from build123d import *

# Parameters (mm, degrees)
SKETCH1_W                = 55
SKETCH1_H                = 80
BACKPANEL_DEPTH          = 3
SKETCH2_W                = 7.325
SKETCH2_H                = 4
MOTORMOUNT_DEPTH         = 34
SKETCH3_W                = 37
SKETCH3_H                = 80
SIDEPANEL2_DEPTH         = 3
SKETCH4_W                = 37
SKETCH4_H                = 80
SIDEPANEL1_DEPTH         = 3
MOTORSUPPORTANGLES_DEPTH = 34
MOTORHOLESSET1_REACH     = 92.957
SKETCH5_R                = 1.515
MOTORHOLESSET2_REACH     = 92.957
SKETCH5_3_R              = 1.515
SKETCH7_W                = 61
SKETCH7_H                = 37
BOTTOMPLATE_DEPTH        = 3
SKETCH8_W                = 61
SKETCH8_H                = 3
CUT_EXTRUDE1_DEPTH       = 37
SKETCH20_W               = 100.196149356
SKETCH20_H               = 67.738241818
SKETCH20_R               = 2
BOSS_EXTRUDE8_DEPTH      = 20
BOSS_EXTRUDE10_DEPTH     = 10
BOSS_EXTRUDE11_DEPTH     = 8
SKETCH24_R               = 1.505
CUT_EXTRUDE6_DEPTH       = 4
SKETCH25_W               = 7.25
SKETCH25_H               = 7.25
BOSS_EXTRUDE12_DEPTH     = 7.25
SKETCH26_R               = 1.515
CUT_EXTRUDE7_DEPTH       = 7.25
CUT_EXTRUDE8_REACH       = 113.941
SKETCH27_W               = 7.325
SKETCH27_H               = 4.500198619
FILLET3_R                = 4.5
SKETCH28_W               = 55
SKETCH28_H               = 16.687272165
CUT_EXTRUDE9_DEPTH       = 3
SKETCH30_W               = 100.196149356
SKETCH30_H               = 67.738241818
CUT_EXTRUDE10_DEPTH      = 10
CHAMFER1_SIZE            = 10
CHAMFER2_SIZE            = 10
CHAMFER3_SIZE            = 10
SKETCH31_R               = 3.5
CUT_EXTRUDE11_DEPTH      = 10
SKETCH32_W               = 49.142704434
SKETCH32_H               = 21.220713278
CUT_EXTRUDE12_DEPTH      = 10
SKETCH33_W               = 25.755482036
SKETCH33_H               = 3
CUT_EXTRUDE13_DEPTH      = 10


with BuildPart() as part:
    # Sketch1 → BackPanel (new body)
    with BuildSketch(Plane.XY):
        with Locations((27.5, 40)):
            Rectangle(SKETCH1_W, SKETCH1_H)
    extrude(amount=BACKPANEL_DEPTH)

    # Sketch2 → MotorMount (add)
    with BuildSketch(Plane.XY.offset(3)):
        with Locations((3.6625, 18.5)):
            Rectangle(SKETCH2_W, SKETCH2_H)
        with Locations((51.3375, 18.5)):
            Rectangle(SKETCH2_W, SKETCH2_H)
    extrude(amount=MOTORMOUNT_DEPTH)

    # Sketch3 → SidePanel2 (add)
    with BuildSketch(Plane.ZY):
        with Locations((18.5, 40)):
            Rectangle(SKETCH3_W, SKETCH3_H)
    extrude(amount=SIDEPANEL2_DEPTH)

    # Sketch4 → SidePanel1 (add)
    with BuildSketch(Plane(origin=(55, 0, 0), x_dir=(0, 0, -1), z_dir=(1, 0, 0))):
        with Locations((-18.5, 40)):
            Rectangle(SKETCH4_W, SKETCH4_H)
    extrude(amount=SIDEPANEL1_DEPTH)

    # Sketch6 → MotorSupportAngles (add)
    with BuildSketch(Plane.XY.offset(37)):
        Polygon((7.325, 16.5), (0, 3.812727835), (0, 16.5), align=None)
        Polygon((47.675, 16.5), (55, 16.5), (55, 3.812727835), align=None)
    extrude(amount=-MOTORSUPPORTANGLES_DEPTH)

    # MotorHolesSet1: up to this plane
    motorholesset1_end = Plane(origin=(7.325, 16.5, -11.65), z_dir=(0.866025403784438, -0.5000000000000012, 0))
    # Sketch5 → MotorHolesSet1 (cut, up to the surface)
    with BuildSketch(Plane(origin=(0, 20.5, 0), x_dir=(1, 0, 0), z_dir=(0, 1, 0)), mode=Mode.PRIVATE) as motorholesset1_sk1:
        with Locations(Location((3.2, -15.1, 0), (0, 0, 270))):
            Circle(SKETCH5_R)
    motorholesset1_tool1 = split(extrude(motorholesset1_sk1.sketch, amount=-MOTORHOLESSET1_REACH, mode=Mode.PRIVATE), bisect_by=motorholesset1_end, keep=Keep.BOTH, mode=Mode.PRIVATE)
    add(motorholesset1_tool1.solids().sort_by_distance((3.2, 20.5, 15.1))[0], mode=Mode.SUBTRACT)
    # Sketch5 → MotorHolesSet1 (cut, up to the surface)
    with BuildSketch(Plane(origin=(0, 20.5, 0), x_dir=(1, 0, 0), z_dir=(0, 1, 0)), mode=Mode.PRIVATE) as motorholesset1_sk2:
        with Locations(Location((3.2, -24.9, 0), (0, 0, 270))):
            Circle(SKETCH5_R)
    motorholesset1_tool2 = split(extrude(motorholesset1_sk2.sketch, amount=-MOTORHOLESSET1_REACH, mode=Mode.PRIVATE), bisect_by=motorholesset1_end, keep=Keep.BOTH, mode=Mode.PRIVATE)
    add(motorholesset1_tool2.solids().sort_by_distance((3.2, 20.5, 24.9))[0], mode=Mode.SUBTRACT)

    # MotorHolesSet2: up to this plane
    motorholesset2_end = Plane(origin=(55, 3.812727835, -11.65), z_dir=(-0.866025403784438, -0.5000000000000011, 0))
    # Sketch5<3> → MotorHolesSet2 (cut, up to the surface)
    with BuildSketch(Plane(origin=(0, 20.5, 0), x_dir=(1, 0, 0), z_dir=(0, 1, 0)), mode=Mode.PRIVATE) as motorholesset2_sk1:
        with Locations(Location((51.8, -15.1, 0), (0, 0, 270))):
            Circle(SKETCH5_3_R)
    motorholesset2_tool1 = split(extrude(motorholesset2_sk1.sketch, amount=-MOTORHOLESSET2_REACH, mode=Mode.PRIVATE), bisect_by=motorholesset2_end, keep=Keep.BOTH, mode=Mode.PRIVATE)
    add(motorholesset2_tool1.solids().sort_by_distance((51.8, 20.5, 15.1))[0], mode=Mode.SUBTRACT)
    # Sketch5<3> → MotorHolesSet2 (cut, up to the surface)
    with BuildSketch(Plane(origin=(0, 20.5, 0), x_dir=(1, 0, 0), z_dir=(0, 1, 0)), mode=Mode.PRIVATE) as motorholesset2_sk2:
        with Locations(Location((51.8, -24.9, 0), (0, 0, 270))):
            Circle(SKETCH5_3_R)
    motorholesset2_tool2 = split(extrude(motorholesset2_sk2.sketch, amount=-MOTORHOLESSET2_REACH, mode=Mode.PRIVATE), bisect_by=motorholesset2_end, keep=Keep.BOTH, mode=Mode.PRIVATE)
    add(motorholesset2_tool2.solids().sort_by_distance((51.8, 20.5, 24.9))[0], mode=Mode.SUBTRACT)

    # Sketch7 → BottomPlate (add)
    with BuildSketch(Plane.XZ):
        with Locations((27.5, 18.5)):
            Rectangle(SKETCH7_W, SKETCH7_H)
    extrude(amount=BOTTOMPLATE_DEPTH)

    # Sketch8 → Cut-Extrude1 (cut)
    with BuildSketch(Plane.XY.offset(37)):
        with Locations((27.5, -1.5)):
            Rectangle(SKETCH8_W, SKETCH8_H)
    extrude(amount=-CUT_EXTRUDE1_DEPTH, mode=Mode.SUBTRACT)



with BuildPart() as body_2:
    # Sketch20 → Boss-Extrude8 (new body)
    with BuildSketch(Plane(origin=(0, -30, 0), x_dir=(-1, 0, 0), z_dir=(0, -1, 0))):
        with Locations((-27.5, -20.61971831)):
            Rectangle(SKETCH20_W, SKETCH20_H)
        with Locations(Location((8, -44.61971831, 0), (0, 0, 90))):
            Circle(SKETCH20_R, mode=Mode.SUBTRACT)
        with Locations(Location((-63, -44.61971831, 0), (0, 0, 90))):
            Circle(SKETCH20_R, mode=Mode.SUBTRACT)
        with Locations(Location((-63, 3.38028169, 0), (0, 0, 90))):
            Circle(SKETCH20_R, mode=Mode.SUBTRACT)
        with Locations(Location((8, 3.38028169, 0), (0, 0, 90))):
            Circle(SKETCH20_R, mode=Mode.SUBTRACT)
    extrude(amount=-BOSS_EXTRUDE8_DEPTH)


with BuildPart() as part_1:
    add(part.part)

    add(body_2.part)  # Boss-Extrude10 merges body 2
    # Sketch21 → Boss-Extrude10 (add)
    with BuildSketch(Plane.XZ):
        Polygon((-3, 0), (58, 0), (58, 37), (55, 37), (55, 3), (0, 3), (0, 37), (-3, 37), align=None)
    extrude(amount=BOSS_EXTRUDE10_DEPTH)

    # Sketch22 → Boss-Extrude11 (add)
    with BuildSketch(Plane.XY.offset(3)):
        Polygon((0, 76.85), (7, 76.85), (7, 73.35), (0, 66.35), align=None)
        Polygon((55, 76.85), (55, 66.35), (48, 73.35), (48, 76.85), align=None)
    extrude(amount=BOSS_EXTRUDE11_DEPTH)

    # Sketch24 → Cut-Extrude6 (cut)
    with BuildSketch(Plane(origin=(0, 76.85, 0), x_dir=(1, 0, 0), z_dir=(0, 1, 0))):
        with Locations(Location((3.5, -7, 0), (0, 0, 180))):
            Circle(SKETCH24_R)
        with Locations(Location((51.5, -7, 0), (0, 0, 180))):
            Circle(SKETCH24_R)
    extrude(amount=-CUT_EXTRUDE6_DEPTH, mode=Mode.SUBTRACT)

    # Sketch25 → Boss-Extrude12 (add)
    with BuildSketch(Plane(origin=(0, -10, 0), x_dir=(1, 0, 0), z_dir=(0, 1, 0))):
        with Locations((3.625, -30.375)):
            Rectangle(SKETCH25_W, SKETCH25_H)
        with Locations((51.375, -30.375)):
            Rectangle(SKETCH25_W, SKETCH25_H)
    extrude(amount=BOSS_EXTRUDE12_DEPTH)

    # Sketch26 → Cut-Extrude7 (cut)
    with BuildSketch(Plane.XY.offset(34)):
        with Locations((3.625, -6.375)):
            Circle(SKETCH26_R)
        with Locations((51.375, -6.375)):
            Circle(SKETCH26_R)
    extrude(amount=-CUT_EXTRUDE7_DEPTH, mode=Mode.SUBTRACT)

    # Cut-Extrude8: up to this plane
    cut_extrude8_end = Plane(origin=(7.325, 16.5, -11.65), z_dir=(0.866025403784438, -0.5000000000000012, 0))
    # Sketch27 → Cut-Extrude8 (cut, up to the surface)
    with BuildSketch(Plane(origin=(0, 20.5, 0), x_dir=(1, 0, 0), z_dir=(0, 1, 0)), mode=Mode.PRIVATE) as cut_extrude8_sk1:
        with Locations((3.6625, -19.611135977)):
            Rectangle(SKETCH27_W, SKETCH27_H)
    cut_extrude8_tool1 = split(extrude(cut_extrude8_sk1.sketch, amount=-CUT_EXTRUDE8_REACH, mode=Mode.PRIVATE), bisect_by=cut_extrude8_end, keep=Keep.BOTH, mode=Mode.PRIVATE)
    add(cut_extrude8_tool1.solids().sort_by_distance((3.6625, 20.5, 19.611136))[0], mode=Mode.SUBTRACT)

    # Fillet3
    fillet3_edges = [part_1.edges().sort_by_distance(p)[0] for p in [
        (48, 75.1, 11),
    ]]
    fillet(fillet3_edges, radius=FILLET3_R)

    # Sketch28 → Cut-Extrude9 (cut)
    with BuildSketch(Plane.XY.offset(37)):
        with Locations((27.5, 12.156363918)):
            Rectangle(SKETCH28_W, SKETCH28_H)
    extrude(amount=-CUT_EXTRUDE9_DEPTH, mode=Mode.SUBTRACT)

    # Sketch30 → Cut-Extrude10 (cut)
    with BuildSketch(Plane.XZ.offset(30)):
        with Locations((27.5, 20.61971831)):
            Rectangle(SKETCH30_W, SKETCH30_H)
    extrude(amount=-CUT_EXTRUDE10_DEPTH, mode=Mode.SUBTRACT)

    # Chamfer1
    chamfer1_edges = [part_1.edges().sort_by_distance(p)[0] for p in [
        (-3, -10, 18.5),
    ]]
    chamfer(chamfer1_edges, length=CHAMFER1_SIZE)

    # Chamfer2
    chamfer2_edges = [part_1.edges().sort_by_distance(p)[0] for p in [
        (58, -10, 18.5),
    ]]
    chamfer(chamfer2_edges, length=CHAMFER2_SIZE)

    # Chamfer3
    # the kernel refuses this chamfer: 10 mm, written as the material it adds along each edge
    with BuildSketch(Plane(origin=(-38.71682988, -10, 0), x_dir=(0, -0.027495876610586317, -0.9996219169112968), z_dir=(1, 0, 0))) as chamfer3_piece_1_section:
        Polygon((CHAMFER3_SIZE * 0.999621916911, CHAMFER3_SIZE * 0.0274958766106), (-CHAMFER3_SIZE * 0.0274958766106, CHAMFER3_SIZE * 0.999621916911), (0, 0), align=None)
    chamfer3_piece_1 = extrude(amount=132.433659759, mode=Mode.PRIVATE)
    chamfer3_piece_1 = split(chamfer3_piece_1, bisect_by=Plane(origin=(-8.165213201, -5.165213201, -8.521451905), z_dir=(0.7071067811865476, -0.7071067811865476, 0)), keep=Keep.TOP, mode=Mode.PRIVATE)
    chamfer3_piece_1 = chamfer3_piece_1 - Plane(origin=(-8, -8.616619282, -3.38028169), x_dir=(0, 0, -1), z_dir=(0, -1, 0)) * Cylinder(2, 305, mode=Mode.PRIVATE)
    chamfer3_piece_1 = split(chamfer3_piece_1, bisect_by=Plane(origin=(-3, -8.616619282, -8.521451905), z_dir=(-1, 0, 0)), keep=Keep.TOP, mode=Mode.PRIVATE)
    add(chamfer3_piece_1)
    with BuildSketch(Plane(origin=(-38.71682988, -10, 0), x_dir=(0, -0.027495876610586317, -0.9996219169112968), z_dir=(1, 0, 0))) as chamfer3_piece_2_section:
        Polygon((CHAMFER3_SIZE * 0.999621916911, CHAMFER3_SIZE * 0.0274958766106), (-CHAMFER3_SIZE * 0.0274958766106, CHAMFER3_SIZE * 0.999621916911), (0, 0), align=None)
    chamfer3_piece_2 = extrude(amount=132.433659759, mode=Mode.PRIVATE)
    chamfer3_piece_2 = split(chamfer3_piece_2, bisect_by=Plane(origin=(-3, -6.7021107, -3.297961008), z_dir=(1, 0, 0)), keep=Keep.TOP, mode=Mode.PRIVATE)
    chamfer3_piece_2 = split(chamfer3_piece_2, bisect_by=Plane(origin=(58, -6.7021107, -3.297961008), z_dir=(-1, 0, 0)), keep=Keep.TOP, mode=Mode.PRIVATE)
    add(chamfer3_piece_2)
    with BuildSketch(Plane(origin=(-38.71682988, -10, 0), x_dir=(0, -0.027495876610586317, -0.9996219169112968), z_dir=(1, 0, 0))) as chamfer3_piece_3_section:
        Polygon((CHAMFER3_SIZE * 0.999621916911, CHAMFER3_SIZE * 0.0274958766106), (-CHAMFER3_SIZE * 0.0274958766106, CHAMFER3_SIZE * 0.999621916911), (0, 0), align=None)
    chamfer3_piece_3 = extrude(amount=132.433659759, mode=Mode.PRIVATE)
    chamfer3_piece_3 = split(chamfer3_piece_3, bisect_by=Plane(origin=(64.879020319, -6.879020319, -8.521451905), z_dir=(-0.7071067811865476, -0.7071067811865476, 0)), keep=Keep.TOP, mode=Mode.PRIVATE)
    chamfer3_piece_3 = chamfer3_piece_3 - Plane(origin=(63, -8.616619283, -3.38028169), x_dir=(0, 0, -1), z_dir=(0, -1, 0)) * Cylinder(2, 305, mode=Mode.PRIVATE)
    chamfer3_piece_3 = split(chamfer3_piece_3, bisect_by=Plane(origin=(58, -8.616619283, -8.521451905), z_dir=(1, 0, 0)), keep=Keep.TOP, mode=Mode.PRIVATE)
    add(chamfer3_piece_3)

    # Sketch31 → Cut-Extrude11 (cut)
    with BuildSketch(Plane(origin=(0, -10, 0), x_dir=(1, 0, 0), z_dir=(0, 1, 0))):
        with Locations(Location((63, 3.38028169, 0), (0, 0, 64.100886192))):
            Circle(SKETCH31_R)
        with Locations(Location((-8, 3.38028169, 0), (0, 0, 115.899113808))):
            Circle(SKETCH31_R)
    extrude(amount=CUT_EXTRUDE11_DEPTH, mode=Mode.SUBTRACT)

    # Sketch32 → Cut-Extrude12 (cut)
    with BuildSketch(Plane(origin=(0, -10, 0), x_dir=(1, 0, 0), z_dir=(0, 1, 0))):
        with Locations((27.5, -14.875)):
            Rectangle(SKETCH32_W, SKETCH32_H)
    extrude(amount=-CUT_EXTRUDE12_DEPTH, mode=Mode.SUBTRACT)

    # Sketch33 → Cut-Extrude13 (cut)
    with BuildSketch(Plane(origin=(0, 80, 0), x_dir=(1, 0, 0), z_dir=(0, 1, 0))):
        with Locations((27.5, -1.5)):
            Rectangle(SKETCH33_W, SKETCH33_H)
    extrude(amount=-CUT_EXTRUDE13_DEPTH, mode=Mode.SUBTRACT)


solid = part_1.part
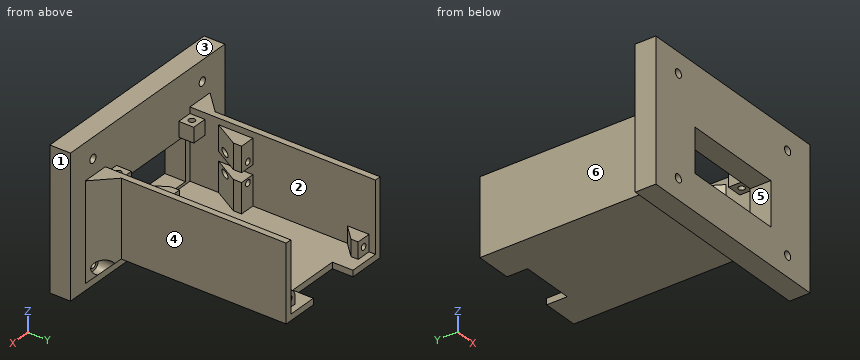
Can you work these out from the model? Positions are in its coordinate system, mm. Face numbers are marked on the shaded views. A direction names the side the tool comes from. Coordinates: 2 decimals unless noted, no trailing zeros. Write each loop counter-clockwise with the first axis right and the second up, starting at its lowest first coordinate (ties: lowest second). Pieces come first, ordered by that corner, then holes.
Q1. Which directions (+Z, -Z, +X, -X, +Y, -Y) give clear straight access to the entire face, cutting with the end or side of a thin tool? Please do the marked faces 4, 5 and 6.
Results found:
face 4: +Z, -Z, +X, +Y
face 5: -Y
face 6: +Z, -Z, -X, +Y
Q2. Imagine slicing it at A-A, the plane x = 45. List the corners of the cut face in (y, z) for me.
Results found:
outline: (-20, -13.25) - (-10, -13.25) - (-10, -10) - (0, 0) - (80, 0) - (80, 3) - (-10, 3) - (-10, 4.26) - (-20, 4.26) - close; (-20, 25.49) - (-10, 25.49) - (-10, 54.49) - (-20, 54.49) - close
Q3. Imagine slicing it at C-C, the plane x = 63. List the corners of the cut face in (y, z) for me.
Results found:
outline: (-20, -13.25) - (-10, -13.25) - (-10, -10) - (-6.88, -6.88) - (-10, -6.88) - (-10, -5.38) - (-20, -5.38) - close; (-20, -1.38) - (-10, -1.38) - (-10, 0.12) - (-5, 0.12) - (-5, 37) - (-10, 37) - (-10, 42.62) - (-20, 42.62) - close; (-20, 46.62) - (-10, 46.62) - (-10, 54.49) - (-20, 54.49) - close
Q4. Imagine slicing it at D-D, the plane z = -8.5. List the corners of the cut face in (x, y) for me, plus the area to 3 significant figures.
Results found:
outline: (-22.6, -20) - (77.6, -20) - (77.6, -10) - (68, -10) - (66.5, -8.5) - (-11.5, -8.5) - (-13, -10) - (-22.6, -10) - close
area: 1,120 mm2
Q5. Please list where these lines run through material, in increasing order: L1, parallel to X at y = 17, z = 15 (3 decimals); L2, parallel to Z at x = 3.2, y = 16 (3 decimals); L3, parallel to X at y = -13.5, z = 6.
Results found:
L1: x = -3 to 1.688, 4.712 to 7.325, 47.675 to 50.288, 53.312 to 58
L2: z = 0 to 13.585, 16.615 to 17.361, 21.861 to 23.385, 26.415 to 34
L3: x = -22.6 to 2.93, 52.07 to 77.6
Q6. Imagine slicing it at B-B, the plane y = 44. List the corners of the cut face in (x, z) for me.
Results found:
outline: (-3, 0) - (58, 0) - (58, 37) - (55, 37) - (55, 3) - (0, 3) - (0, 37) - (-3, 37) - close
Q7. For P1, Ø6, axis at y = -1.5, z = 13.5, coming from the -X side; P2, Ø2.5, axis at x = 3.5, z = 7, coming from the -Y side; P3, Ø6, axis at x = 4.5, y = -6.5, coming from the -Z side; P4, Ø2, axis at x = 50, y = 10, coming from the +Z side, each with a flat end and sliding along its axis, tell me the tip position at first contact or that it passes through.
Results found:
P1: stops at x = -7.5
P2: stops at y = -20
P3: stops at z = -9.5
P4: stops at z = 3
Q8. If we mould it in two halves opening along X, with no side actions, what happens to the marked faces 1, 2 and 3? For each: +X half, -X half, draft (parallel to the pull), parting line (faces both ways), or undercut.
Results found:
face 1: +X half
face 2: undercut
face 3: draft
